Autodesk Inventor part; units mm, degrees
ref_plane "YZ Plane" through (0, 0, 0) normal (1, 0, 0) x (0, 1, 0)
ref_plane "XZ Plane" through (0, 0, 0) normal (0, 1, 0) x (-1, 0, 0)
ref_plane "XY Plane" through (0, 0, 0) normal (0, 0, 1) x (1, 0, 0)
sketch "Sketch1" plane through (0, 0, 0) normal (0, 0, 1) x (1, 0, 0)
  circle A0 centre (0, 0) radius 10
  dimension "d0" = 20
extrude "Extrusion1" add sketch "Sketch1" along normal blind 20
sketch "Sketch2" plane through (0, 0, 20) normal (0, 0, 1) x (1, 0, 0)
  circle A0 centre (0, 0) radius 10
  line L0 (0, 10) -> (0, -10) construction
  line L1 (3, 9.5394) -> (3, -9.5394)
  line L2 (-3, 9.5394) -> (-3, -9.5394)
  arc A1 (-3, -9.5394) -> (3, -9.5394) centre (0, 0) ccw
  arc A2 (3, 9.5394) -> (-3, 9.5394) centre (0, 0) ccw
  dimension "d3" = 3
  dimension "d4" = 3
extrude "Extrusion2" add sketch "Sketch2" along normal blind 5 contours L1 A0 L2
hole "Hole1" at (0, 0, 0) direction (0, 0, 1) diameter 4.2 end through all
properties part number "Ender 5 Foot Spacer"
Read the model definition and answer for the solid it produces. Units are mm, in the model's axes. A direction names the side the tool comes from. Round coordinates to 2 decimals unless told otherwise and drop trailing zeros. Write each loop counter-clockwise with the first axis right and the second up, starting at its lowest first coordinate (ties: lowest second). Pieces come first, ordered by that corner, then holes. Notation, with made-up numbers: (33, -30.5) - (53, -30.5) arc R18 ccw to (53, -24.5) - close; hole circle Ø11 at (51.5, 67). An arc over 180 degrees is marked (long way). Use CSV: the item, a comma, the result in double quotes.
Q1. Each of these flat-tipped pins is pushed along its axis until it touches: pin 1 Ø1.5 at (x, z) = (3, 8) entering from +Y; pin 2 Ø4 at (y, z) = (-7.5, 8.5) entering from -X; pin 3 Ø3 at (x, z) = (-5, 14) entering from -Y; pin 4 Ø2 at (x, z) = (-5.5, 22) entering from -Y. Where does it stop, or does it pass through?
Values:
pin 1,"stops at y = 9.74"
pin 2,"stops at x = -8.35"
pin 3,"stops at y = -9.37"
pin 4,"passes through"
Q2. Find section B-B, the plane x = 0. Write down the section's boundary in (y, z).
Values:
outline,"(-10, 0) - (-2.1, 0) - (-2.1, 25) - (-10, 25) - close; (2.1, 0) - (10, 0) - (10, 25) - (2.1, 25) - close"
Q3. A tool of negligible diameter and unlimited length cuts with its end or side. For faces 1 (the flat face through (-6, 0, 20)), 2 (the flat face through (0, 2.4, 25)), 3 (the flat face through (6, 0, 20)), from which of +Z, -Z, +X, -X, +Y, -Y can it reach the whole face along a straight path? Write none if from no direction.
Values:
face 1,"+Z, -X, +Y, -Y"
face 2,"+Z, +X, -X, +Y, -Y"
face 3,"+Z, +X, +Y, -Y"
Q4. Determine the mould class of faces 4 (the flat face through (-0.1, 2.4, 0)), 5 (the flat face through (3, 0, 22)), 6 (the cylindrical face through (-0.631, 2.003, 12.675)) for opening direction X: +X half, -X half, draft (parallel to the pull), parting line (faces both ways), or undercut.
Values:
face 4,"draft"
face 5,"+X half"
face 6,"undercut"
Q5. Straight lines are drawn through the part: line 1 along X through (y, z) = (0, 7); line 2 along Z through (x, y) = (5, -7). For each, find the intervals that lie inside material, in ascending order.
Values:
line 1,"x = -10 to -2.1, 2.1 to 10"
line 2,"z = 0 to 20"
Q6. Find section D-D, the plane y = 5.75. Write down the section's boundary in (x, z).
Values:
outline,"(-8.18, 0) - (8.18, 0) - (8.18, 20) - (3, 20) - (3, 25) - (-3, 25) - (-3, 20) - (-8.18, 20) - close"
Q7. Find section A-A, the plane y = 0. Write down the section's boundary in (x, z).
Values:
outline,"(-10, 0) - (-2.1, 0) - (-2.1, 25) - (-3, 25) - (-3, 20) - (-10, 20) - close; (2.1, 0) - (10, 0) - (10, 20) - (3, 20) - (3, 25) - (2.1, 25) - close"
Q8. Find section C-C, the plane z = 20.5. Write down the section's boundary in (x, y), then the cut area to 3 significant figures.
Values:
outline,"(-3, -9.54) arc R10 ccw to (3, -9.54) - (3, 9.54) arc R10 ccw to (-3, 9.54) - close; hole circle Ø4.2 at (0, 0)"
area,"104 mm²"
